from build123d import *

# Parameters (mm, degrees)
F0_R     = 1.5
F1_DEPTH = 9.525
F2_R     = 1.25
F3_DEPTH = 25.401


# Not quite as in the source:
# - a length typed as a fraction of an inch, garbled in the dataset ("3 / 203.2 mm" for 3/8 in), is restored


with BuildPart() as f1:
    # F0 (on Top) → F1 (new body)
    with BuildSketch(Plane.XY):
        with BuildLine():
            Line((-7, -12.7), (7, -12.7))
            Line((7, -12.7), (7, 12.7))
            Line((7, 12.7), (-7, 12.7))
            Line((-7, 12.7), (-7, 7.2))
            Line((-7, 7.2), (-0.0847406698, 7.2))
            ThreePointArc((-0.0847406698, 7.2), (6.125, 6.7), (-0.0847406698, 6.2))
            Line((-0.0847406698, 6.2), (-7, 6.2))
            Line((-7, 6.2), (-7, -12.7))
        make_face()
        with Locations((3, -7.3)):
            Circle(F0_R, mode=Mode.SUBTRACT)
    extrude(amount=F1_DEPTH)

    # F2 (on face) → F3 (cut, through all)
    with BuildSketch(Plane(origin=(0, 12.7, 0), x_dir=(-1, 0, 0), z_dir=(0, 1, 0))):
        with Locations((3.5423703349, 4.7625)):
            Circle(F2_R)
    extrude(amount=-F3_DEPTH, mode=Mode.SUBTRACT)


solid = f1.part
The listing builds one solid part. Answer for the finished solid, in the listing's coordinates (mm). A direction names the side the tool comes from. Coordinates: 2 decimals unless noted, no trailing zeros. Order: outer loops, then holes, each group sorted by start corner. A loop starts at its lowest first (then second) coordinate and runs counter-clockwise, first axis right, second up.
Q1. For a pull along X with two mould halves and no side action, classify faces 1 (the face through (0, 12.7, 5)), 2 (the face through (2.675, -8.764, 4.696)), 3 (the face through (7, 0, 5)) as pulls with the +X half, pulls with the -X half, needs draft (parallel to the pull), parting line crosses it, or undercut.
Q2. A cutting plane is placed at C-C, the plane x = 3. Write down the section's boundary in (y, z) (3 decimals), and give its area (3 significant figures).
Q3. A cutting plane is placed at B-B, the plane y = -7.3. State how many separate pieces and enclosed holes the cut face has, and give its area (3 significant figures).
Q4. Consider line 1 (Y direction, x = 3, z = 5) (3 decimals); line 2 (Y direction, x = -2.5, z = 4); line 3 (Y direction, x = 3.5, z = 7). Determine where each line is inside the solid, lowest interval first.
Q5. Given P1, Ø2, axis at x = -3.54, z = 4.76, coming from the +Y side, flat-ended and moving along its own axis, determine where the tip first touches the part or whether it passes through.
Q6. A cutting plane is placed at D-D, the plane z = 7.5. Write down the section's boundary in (x, y) (3 decimals).
Q7. A cutting plane is placed at A-A, the plane x = -1. Write down the section's boundary in (y, z) (3 decimals), and give its area (3 significant figures).
Q8. Which of the six approach directions +Z, -Z, +X, -X, +Y, -Y give full straight-line access (tool end or side, diameter ignored) to faces 4 (the face through (-4.4, 7.2, 3.6)), 5 (the face through (-7, -3, 5))?
Answers follow:
1. face 1: needs draft
1. face 2: undercut
1. face 3: pulls with the +X half
2. outline: (-12.7, 0) - (-8.8, 0) - (-8.8, 9.525) - (-12.7, 9.525) - close; (-5.8, 0) - (3.575, 0) - (3.575, 9.525) - (-5.8, 9.525) - close; (9.825, 0) - (12.7, 0) - (12.7, 9.525) - (9.825, 9.525) - close
2. area: 154 mm2
3. separate pieces: 2
3. enclosed holes: 1
3. area: 99.9 mm2
4. line 1: y = -12.7 to -8.8, -5.8 to 3.575, 9.825 to 12.7
4. line 2: y = -12.7 to 6.2, 7.2 to 12.7
4. line 3: y = -12.7 to -8.71, -5.89 to 3.62, 9.78 to 12.7
5. P1: passes through
6. outline: (-7, -12.7) - (7, -12.7) - (7, 12.7) - (-7, 12.7) - (-7, 7.2) - (-0.085, 7.2) arc R3.125 cw (long way) to (-0.085, 6.2) - (-7, 6.2) - close; hole circle Ø3 at (3, -7.3)
7. outline: (-12.7, 0) - (6.2, 0) - (6.2, 9.525) - (-12.7, 9.525) - close; (7.2, 0) - (12.7, 0) - (12.7, 9.525) - (7.2, 9.525) - close
7. area: 232 mm2
8. face 4: +Z, -Z, -X
8. face 5: +Z, -Z, -X, +Y, -Y
